Here's how the part is built. I have some questions about the finished solid (model axes, mm). A direction names the side the tool comes from. Round coordinates to 2 decimals unless told otherwise and drop trailing zeros. Write each loop counter-clockwise with the first axis right and the second up, starting at its lowest first coordinate (ties: lowest second). Pieces come first, ordered by that corner, then holes. Notation, with made-up numbers: (71, 44) -> (109, 44) arc R25 ccw to (109, 58) -> close; hole circle Ø11 at (71.5, 18.25). An arc over 180 degrees is marked (long way). Put each result on its own line as item: value. Start each with the question number.
1) I want a section at C-C, the plane y = -7.5. List the corners of the cut face in (x, z) for me.
2) If I drill on line 1 along Z through (x, y) = (6.5, 5.75); line 2 along Z through (x, y) = (2.5, 1); line 3 along Y through (x, z) = (-8.25, 51.95), over which ranges is the centre line in solid material (lowest first)? Write a range as [from, to].
3) I want a section at D-D, the plane z = 40. List the corners of the cut face in (x, y) for me.
4) Will these pins go through, and if not, where does the flat tip stop? P1, Ø6, axis at x = 7.5, z = 27, coming from the -Y side; P2, Ø8, axis at y = 6.5, z = 14.5, coming from the +X side; P3, Ø6, axis at x = -7.5, z = 14, coming from the +Y side.
5) I want a section at A-A, the plane x = 0. List the corners of the cut face in (y, z) for me, then the cut area to 3 significant figures.
6) Which directions (+Z, -Z, +X, -X, +Y, -Y) give clear straight access to the entire face, cutting with the end or side of a thin tool? Please do faces 5 (the cylindrical face through (3.233, -1.341, 54.232)), 6 (the cylindrical face through (2.02, -3.16, -0.49)), 7 (the flat face through (0, 1, 61)).
7) I want a section at B-B, the plane z = 51. List the corners of the cut face in (x, y) for me, then the cut area to 3 significant figures.
8) We'd pull the mould along X, two halves only. Please class faces 1 (the flat face through (-8, 0, 48)), 2 (the flat face through (0, 0, -2)), 3 (the cylindrical face through (11.923, 3.755, 41.339)), 4 (the cylindrical face through (-9.75, 0.07, 50.54)): released by +X, released by -X, zero draft, split by the parting line, or undercut.
from build123d import *

# Parameters (mm, degrees)
SKETCH1_R           = 12.25
BOSS_EXTRUDE1_DEPTH = 30
SKETCH2_R           = 12.5
BOSS_EXTRUDE2_DEPTH = 23
CUT_EXTRUDE1_DEPTH  = 5
SKETCH3_R           = 3.5
BOSS_EXTRUDE3_DEPTH = 2.5
SKETCH4_R           = 2
BOSS_EXTRUDE4_DEPTH = 1.5
BOSS_EXTRUDE5_DEPTH = 8
SKETCH6_R           = 3.75
BOSS_EXTRUDE6_DEPTH = 2
FILLET1_R           = 1


with BuildPart() as part:
    # Sketch1 → Boss-Extrude1 (new body)
    with BuildSketch(Plane.XY):
        Circle(SKETCH1_R)
    extrude(amount=BOSS_EXTRUDE1_DEPTH)

    # Sketch2 → Boss-Extrude2 (add)
    with BuildSketch(Plane.XY.offset(30)):
        Circle(SKETCH2_R)
    extrude(amount=BOSS_EXTRUDE2_DEPTH)

    # Sketch7 → Cut-Extrude1 (cut)
    with BuildSketch(Plane.XY.offset(53)):
        with BuildLine():
            ThreePointArc((-9.75, 0), (-8.25, -1.5), (-6.75, 0))
            Line((-6.75, 0), (-8.25, 0))
            Line((-8.25, 0), (-9.75, 0))
        make_face()
        with BuildLine():
            Line((-8.25, 0), (-6.75, 0))
            ThreePointArc((-6.75, 0), (-8.25, 1.5), (-9.75, 0))
            Line((-9.75, 0), (-8.25, 0))
        make_face()
        with BuildLine():
            ThreePointArc((6.75, 0), (8.25, -1.5), (9.75, 0))
            Line((9.75, 0), (8.25, 0))
            Line((8.25, 0), (6.75, 0))
        make_face()
        with BuildLine():
            Line((8.25, 0), (9.75, 0))
            ThreePointArc((9.75, 0), (8.25, 1.5), (6.75, 0))
            Line((6.75, 0), (8.25, 0))
        make_face()
    extrude(amount=-CUT_EXTRUDE1_DEPTH, mode=Mode.SUBTRACT)

    # Sketch3 → Boss-Extrude3 (add)
    with BuildSketch(Plane.XY.offset(53)):
        Circle(SKETCH3_R)
    extrude(amount=BOSS_EXTRUDE3_DEPTH)

    # Sketch4 → Boss-Extrude4 (add)
    with BuildSketch(Plane.XY.offset(55.5)):
        Circle(SKETCH4_R)
    extrude(amount=BOSS_EXTRUDE4_DEPTH)

    # Sketch5 → Boss-Extrude5 (add)
    with BuildSketch(Plane.XY.offset(57)):
        with BuildLine():
            Line((1.732050808, 1), (-1.732050808, 1))
            ThreePointArc((-1.732050808, 1), (-0.51763809, -1.931851653), (2, 0))
            ThreePointArc((2, 0), (1.931851653, 0.51763809), (1.732050808, 1))
        make_face()
    extrude(amount=BOSS_EXTRUDE5_DEPTH)

    # Sketch6 → Boss-Extrude6 (add)
    with BuildSketch(Plane(origin=(0, 0, 0), x_dir=(-1, 0, 0), z_dir=(0, 0, -1))):
        with Locations(Location((0, 0, 0), (0, 0, 180))):
            Circle(SKETCH6_R)
    extrude(amount=BOSS_EXTRUDE6_DEPTH)

    # Fillet1
    fillet1_edges = [part.edges().sort_by_distance(p)[0] for p in [
        (-3.75, 0, -2),
    ]]
    fillet(fillet1_edges, radius=FILLET1_R)


solid = part.part
Findings:
1. outline: (-10, 30) -> (-9.69, 30) -> (-9.69, 0) -> (9.69, 0) -> (9.69, 30) -> (10, 30) -> (10, 53) -> (-10, 53) -> close
2. line 1: z = [0, 53]
2. line 2: z = [-2, 55.5]
2. line 3: y = [-9.39, -1.5], [1.5, 9.39]
3. outline: circle Ø25 at (0, 0)
4. P1: stops at y = -11.39
4. P2: stops at x = 11.99
4. P3: stops at y = 11.39
5. outline: (-12.5, 30) -> (-12.25, 30) -> (-12.25, 0) -> (-3.75, 0) -> (-3.75, -1) arc R1 ccw to (-2.75, -2) -> (2.75, -2) arc R1 ccw to (3.75, -1) -> (3.75, 0) -> (12.25, 0) -> (12.25, 30) -> (12.5, 30) -> (12.5, 53) -> (3.5, 53) -> (3.5, 55.5) -> (2, 55.5) -> (2, 57) -> (1, 57) -> (1, 65) -> (-2, 65) -> (-2, 55.5) -> (-3.5, 55.5) -> (-3.5, 53) -> (-12.5, 53) -> close
5. area: 1,370 mm2
6. face 5: +Z
6. face 6: -Z
6. face 7: +Z, +X, -X, +Y
7. outline: circle Ø25 at (0, 0); hole circle Ø3 at (-8.25, 0); hole circle Ø3 at (8.25, 0)
7. area: 477 mm2
8. face 1: undercut
8. face 2: zero draft
8. face 3: split by the parting line
8. face 4: undercut
